Could you check a few things on this drawing? It's one solid part, dimensions in mm from its lowest x, y, z. A direction names the side the tool comes from. Coordinates: 2 decimals unless noted, no trailing zeros. Order: outer loops, then holes, each group sorted by start corner. A loop starts at its lowest first (then second) coordinate and runs counter-clockwise, first axis right, second up. Notation, with made-up numbers: (23, 16) -> (45, 16) arc R35 ccw to (45, 52) -> close; hole circle Ø11 at (62, -7). An arc over 180 degrees is marked (long way). Use a Markdown table: item, result. Add a question column.
1. Suppose I cut it at A-A, the plane y = 4. List the corners of the cut face in (x, z) for me.
2. For the marked faces 1 and 2, which set-ups out of +Z, -Z, +X, -X, +Y, -Y let a thin tool reach every point of the face, with its end or its side?
3. We'd pull the mould along X, two halves only. Please class the marked faces 3, 4, 5 and 6: pulls with the +X half, pulls with the -X half, needs draft (parallel to the pull), parting line crosses it, or undercut.
4. For pin 1 Ø10 at (x, z) = (11, 22.5) entering from -Y; pin 2 Ø0.6 at (y, z) = (6.5, 18) entering from +X; pin 3 Ø3 at (x, y) = (9, 2) entering from +Z, each with a flat end and sliding along its axis, tell me the tip position at first contact or that it passes through.
5. If I drill on line 1 along Y through (x, z) = (12, 7); line 2 along X through (y, z) = (1, 18.5); line 3 along Z through (x, y) = (26.5, 3.5), over which ranges is the centre line in solid material (lowest first)? Write a range as from..to.
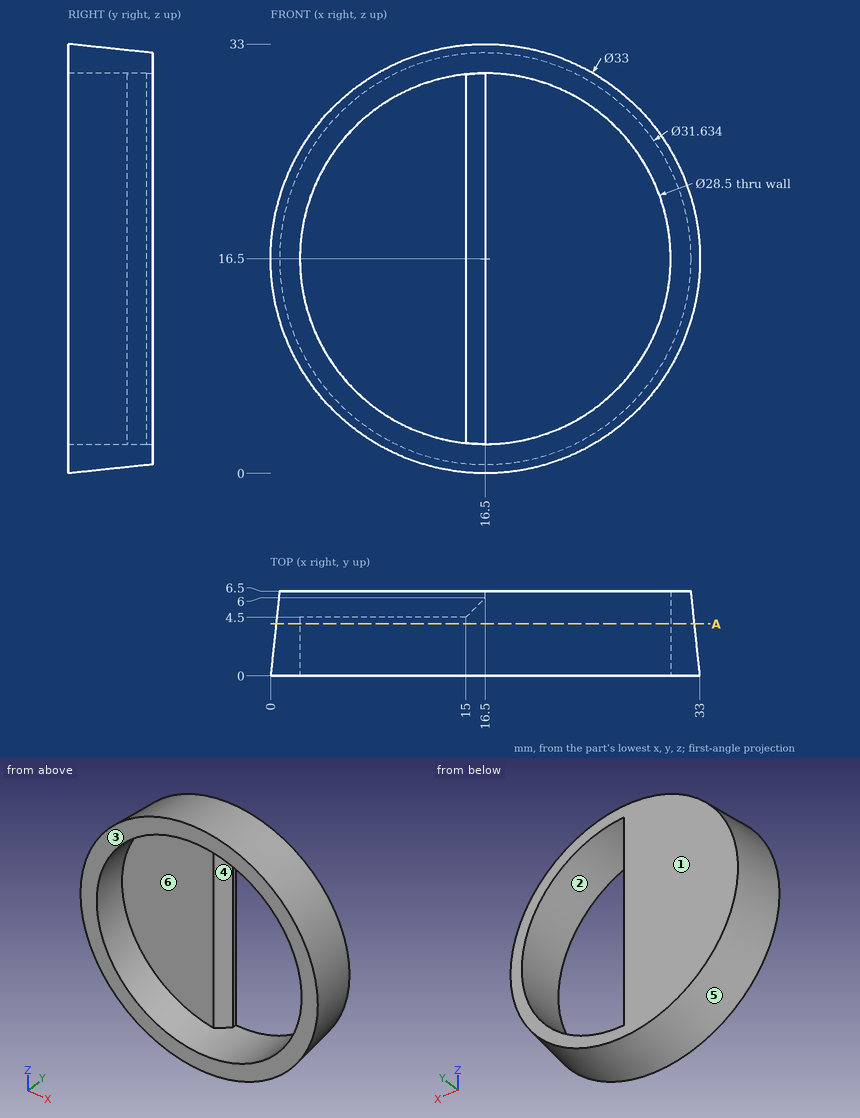
Worked out:
| question | item | result |
|---|---|---|
| 1 | outline | circle Ø32.16 at (16.5, 16.5); hole circle Ø28.5 at (16.5, 16.5) |
| 2 | face 1 | +Z, -Z, +X, -X, +Y |
| 2 | face 2 | -Y |
| 3 | face 3 | needs draft |
| 3 | face 4 | undercut |
| 3 | face 5 | parting line crosses it |
| 3 | face 6 | undercut |
| 4 | pin 1 | stops at y = 4.5 |
| 4 | pin 2 | stops at x = 32.29 |
| 4 | pin 3 | stops at z = 31.67 |
| 5 | line 1 | y = 4.5..6.5 |
| 5 | line 2 | x = 0.23..2.39, 30.61..32.77 |
| 5 | line 3 | z = 3.84..6.35, 26.65..29.16 |
